Source: CAD feature listing. Evaluate the final solid. Frame: model axes, mm. Round coordinates to 2 decimals unless told otherwise and drop trailing zeros. Write each loop counter-clockwise with the first axis right and the second up, starting at its lowest first coordinate (ties: lowest second). Pieces come first, ordered by that corner, then holes. Notation, with made-up numbers: M -34.75,-40 L 21.25,-40 A25 cw 21.25,-10 Z; hole C -20,48.5 d7. An arc over 180 degrees is marked long. Answer in a Markdown table with one row per item.
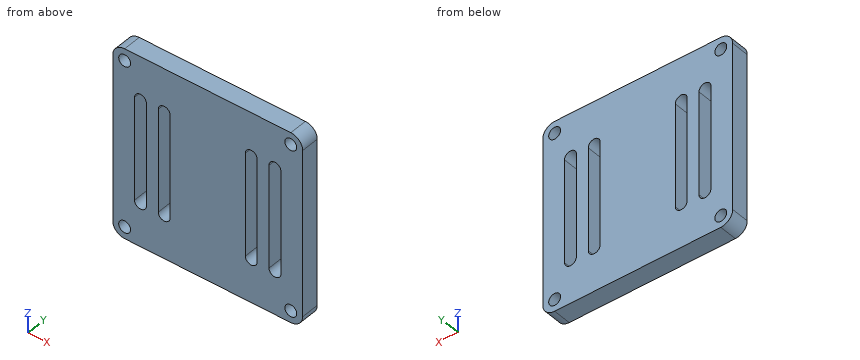
from build123d import *

# Parameters (mm, degrees)
SKETCH3_R           = 1.5
BOSS_EXTRUDE1_DEPTH = 4.572


with BuildPart() as part:
    # Sketch3 → Boss-Extrude1 (new body)
    with BuildSketch(Plane(origin=(0, 0, 0), x_dir=(1, 0, 0), z_dir=(0, 1, 0))):
        with BuildLine():
            Line((3, 0), (45, 0))
            ThreePointArc((45, 0), (47.121320344, 0.878679656), (48, 3))
            Line((48, 3), (48, 45))
            ThreePointArc((48, 45), (47.121320344, 47.121320344), (45, 48))
            Line((45, 48), (3, 48))
            ThreePointArc((3, 48), (0.878679656, 47.121320344), (0, 45))
            Line((0, 45), (0, 3))
            ThreePointArc((0, 3), (0.878679656, 0.878679656), (3, 0))
        make_face()
        with Locations(Location((3, 45, 0), (0, 0, 270))):
            Circle(SKETCH3_R, mode=Mode.SUBTRACT)
        with Locations(Location((3, 3, 0), (0, 0, 90))):
            Circle(SKETCH3_R, mode=Mode.SUBTRACT)
        with Locations(Location((45, 3, 0), (0, 0, 270))):
            Circle(SKETCH3_R, mode=Mode.SUBTRACT)
        with Locations(Location((45, 45, 0), (0, 0, 90))):
            Circle(SKETCH3_R, mode=Mode.SUBTRACT)
        with BuildLine():
            Line((8.5, 37), (8.5, 11))
            ThreePointArc((8.5, 11), (7, 9.5), (5.5, 11))
            Line((5.5, 11), (5.5, 37))
            ThreePointArc((5.5, 37), (7, 38.5), (8.5, 37))
        make_face(mode=Mode.SUBTRACT)
        with BuildLine():
            Line((11.5, 37), (11.5, 11))
            ThreePointArc((11.5, 11), (13, 9.5), (14.5, 11))
            Line((14.5, 11), (14.5, 37))
            ThreePointArc((14.5, 37), (13, 38.5), (11.5, 37))
        make_face(mode=Mode.SUBTRACT)
        with BuildLine():
            Line((36.5, 37), (36.5, 11))
            ThreePointArc((36.5, 11), (35, 9.5), (33.5, 11))
            Line((33.5, 11), (33.5, 37))
            ThreePointArc((33.5, 37), (35, 38.5), (36.5, 37))
        make_face(mode=Mode.SUBTRACT)
        with BuildLine():
            Line((39.5, 37), (39.5, 11))
            ThreePointArc((39.5, 11), (41, 9.5), (42.5, 11))
            Line((42.5, 11), (42.5, 37))
            ThreePointArc((42.5, 37), (41, 38.5), (39.5, 37))
        make_face(mode=Mode.SUBTRACT)
    extrude(amount=BOSS_EXTRUDE1_DEPTH)


solid = part.part
Q1. Section A-A (z = -29.5). Return loops of the section in (x, y), and give its area (3 significant figures).
Solutions:
| item | result |
|---|---|
| outline | M 0,0 L 5.5,0 L 5.5,4.57 L 0,4.57 Z; M 8.5,0 L 11.5,0 L 11.5,4.57 L 8.5,4.57 Z; M 14.5,0 L 33.5,0 L 33.5,4.57 L 14.5,4.57 Z; M 36.5,0 L 39.5,0 L 39.5,4.57 L 36.5,4.57 Z; M 42.5,0 L 48,0 L 48,4.57 L 42.5,4.57 Z |
| area | 165 mm2 |
Q2. Section B-B (x = 13). Return loops of the section in (y, z).
Solutions:
| item | result |
|---|---|
| outline | M 0,-48 L 4.57,-48 L 4.57,-38.5 L 0,-38.5 Z; M 0,-9.5 L 4.57,-9.5 L 4.57,0 L 0,0 Z |
Q3. Section C-C (y = 2.75). State how many separate pieces and enclosed holes the cut face has, and give its area (3 significant figures).
Solutions:
| item | result |
|---|---|
| separate pieces | 1 |
| enclosed holes | 8 |
| area | 1,930 mm2 |
Q4. Material intervals for probe 1 along X at (y, z) = (2.4, -34); probe 2 along X at (y, z) = (1.75, -45); probe 3 along Z at (x, y) = (13, 4.15), sorted ascending.
Solutions:
| item | result |
|---|---|
| probe 1 | x = 0 to 5.5, 8.5 to 11.5, 14.5 to 33.5, 36.5 to 39.5, 42.5 to 48 |
| probe 2 | x = 0 to 1.5, 4.5 to 43.5, 46.5 to 48 |
| probe 3 | z = -48 to -38.5, -9.5 to 0 |
